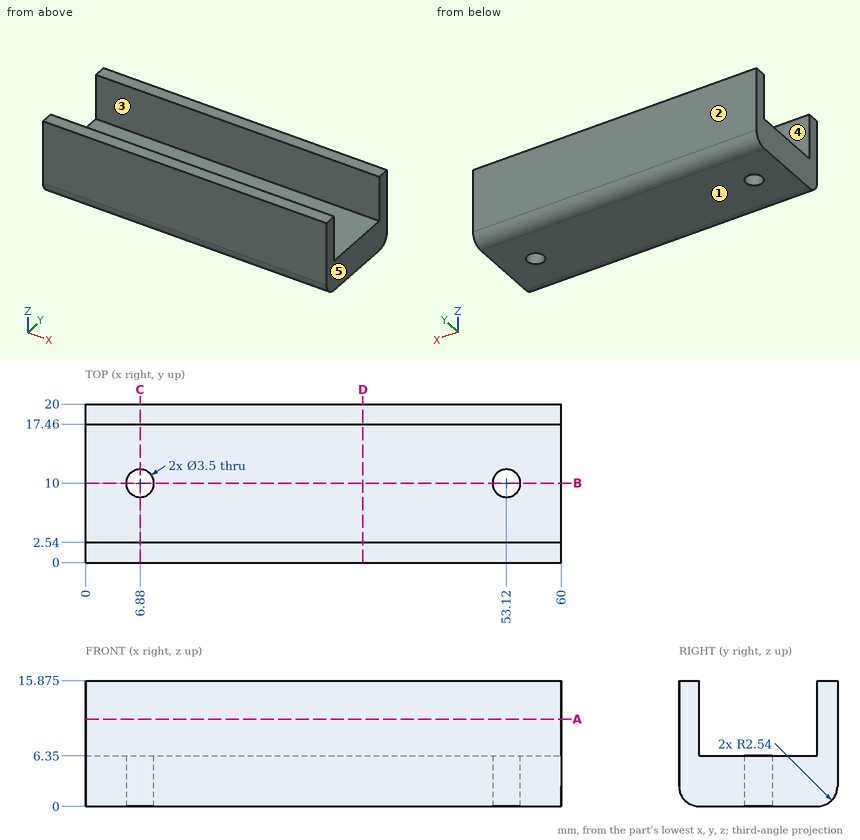
Could you check a few things on this drawing? It's one solid part, dimensions in mm from its lowest x, y, z. A direction names the side the tool comes from. Give positions to 0.01 mm unless a question says otherwise; leave off trailing zeros. Write each loop counter-clockwise with the first axis right and the second up, starting at its lowest first coordinate (ties: lowest second). Pieces come first, ordered by that corner, then holes. Notation, with made-up numbers: (78, 9) -> (112, 9) arc R16 cw to (112, 14) -> close; hole circle Ø9 at (52.25, -12). An arc over 180 degrees is marked (long way). Write item = value, one per line.
(1) Thinking about a two-plate mould opening in Y: for the marked faces 1, 2 and 3, which applies, released by +Y, released by -Y, zero draft, split by the parting line, or undercut?
Worked out:
face_1 = zero draft
face_2 = released by +Y
face_3 = undercut
(2) Suppose I cut it at D-D on x = 35. Write out the boundary of the cut face in (y, z) (3 decimals), then the cut area to 3 significant figures.
Worked out:
outline = (0, 2.54) arc R2.54 ccw to (2.54, 0) -> (17.46, 0) arc R2.54 ccw to (20, 2.54) -> (20, 15.875) -> (17.46, 15.875) -> (17.46, 6.35) -> (2.54, 6.35) -> (2.54, 15.875) -> (0, 15.875) -> close
area = 173 mm^2
(3) I need wall thicknesses on probe 1 along Y at (x, z) = (55, 14.5); probe 2 along Y at (x, z) = (6.88, 5); probe 3 along X at (y, z) = (11.25, 2.25). Which ranges of each line are inside material? Lowest first, please. Write a range as from..to.
Worked out:
probe_1 = 0..2.54, 17.46..20
probe_2 = 0..8.25, 11.75..20
probe_3 = 0..5.66, 8.1..51.9, 54.34..60
(4) Suppose I cut it at C-C on x = 6.88. Write out the boundary of the cut face in (y, z) (3 decimals), then the cut area to 3 significant figures.
Worked out:
outline = (0, 2.54) arc R2.54 ccw to (2.54, 0) -> (8.25, 0) -> (8.25, 6.35) -> (2.54, 6.35) -> (2.54, 15.875) -> (0, 15.875) -> close; (11.75, 0) -> (17.46, 0) arc R2.54 ccw to (20, 2.54) -> (20, 15.875) -> (17.46, 15.875) -> (17.46, 6.35) -> (11.75, 6.35) -> close
area = 150 mm^2
(5) Suppose I cut it at B-B on y = 10. Write out the boundary of the cut face in (x, z).
Worked out:
outline = (0, 0) -> (5.13, 0) -> (5.13, 6.35) -> (0, 6.35) -> close; (8.63, 0) -> (51.37, 0) -> (51.37, 6.35) -> (8.63, 6.35) -> close; (54.87, 0) -> (60, 0) -> (60, 6.35) -> (54.87, 6.35) -> close
(6) Suppose I cut it at A-A on z = 11. Write out the boundary of the cut face in (x, y), then the cut area to 3 significant figures.
Worked out:
outline = (0, 0) -> (60, 0) -> (60, 2.54) -> (0, 2.54) -> close; (0, 17.46) -> (60, 17.46) -> (60, 20) -> (0, 20) -> close
area = 305 mm^2
(7) For the marked faces 4 and 5, which set-ups out of +Z, -Z, +X, -X, +Y, -Y let a thin tool reach every point of the face, with its end or its side?
Worked out:
face_4 = +Z, +X, -X
face_5 = +Z, -Z, +X, +Y, -Y
(8) I'm going to push a flat-ended pin straight in: P1, Ø4.5, axis at x = 18.5, y = 13.5, coming from the +Z side. Where does the tip first touch, or does it pass through?
Worked out:
P1 = 6.35
